from build123d import *

# Parameters (mm, degrees)
AUFSATZ_LINEAR_AUSTRAGEN1_DEPTH      = 9.8
AUFSATZ_LINEAR_AUSTRAGEN1_DEPTH_BACK = 9.8
SKIZZE1_R                            = 9.6
SKIZZE2_R                            = 11.1
AUFSATZ_LINEAR_AUSTRAGEN2_DEPTH      = 1.4
AUFSATZ_LINEAR_START                 = -1.4
SKIZZE3_R                            = 11.1
AUFSATZ_LINEAR_AUSTRAGEN3_DEPTH      = 1.4
SKIZZE4_R                            = 2
SKIZZE4_R_2                          = 3.4
SCHNITT_LINEAR_AUSTRAGEN1_DEPTH      = 1.35
KREISMUSTER1_COUNT                   = 4
SKIZZE9_R                            = 1.5
SCHNITT_LINEAR_AUSTRAGEN2_DEPTH      = 1.2


with BuildPart() as part:
    # Skizze1 → Aufsatz-Linear austragen1 (new, two sides: drawn at the far end of the back side and taken through both)
    with BuildSketch(Plane.XY.offset(-AUFSATZ_LINEAR_AUSTRAGEN1_DEPTH_BACK)):
        Circle(SKIZZE1_R)
    extrude(amount=AUFSATZ_LINEAR_AUSTRAGEN1_DEPTH + AUFSATZ_LINEAR_AUSTRAGEN1_DEPTH_BACK)

    # Skizze2 → Aufsatz-Linear austragen2 (add)
    with BuildSketch(Plane.XY.offset(9.8)):
        Circle(SKIZZE2_R)
    extrude(amount=-AUFSATZ_LINEAR_AUSTRAGEN2_DEPTH)

    # Skizze3 → Aufsatz-Linear austragen3 (add)
    with BuildSketch(Plane(origin=(0, 0, -9.8), x_dir=(-1, 0, 0), z_dir=(0, 0, -1)).offset(AUFSATZ_LINEAR_START)):
        with Locations(Location((0, 0, 0), (0, 0, 180))):
            Circle(SKIZZE3_R)
    extrude(amount=AUFSATZ_LINEAR_AUSTRAGEN3_DEPTH)

    # Skizze4 → Schnitt-Linear austragen1 (cut)
    with BuildSketch(Plane.XY.offset(9.8)):
        with Locations((0, 8.3)):
            Circle(SKIZZE4_R)
        with BuildLine():
            Line((-1.971343548, 8.637349398), (-3.351284031, 0.573493976))
            ThreePointArc((-3.351284031, 0.573493976), (0, 3.4), (3.351284031, 0.573493976))
            Line((3.351284031, 0.573493976), (1.971343548, 8.637349398))
            ThreePointArc((1.971343548, 8.637349398), (1.99282301, 8.469282167), (2, 8.3))
            ThreePointArc((2, 8.3), (-0.169282167, 6.30717699), (-1.971343548, 8.637349398))
        make_face()
        Circle(SKIZZE4_R_2)
    schnitt_linear_austragen1 = extrude(amount=-SCHNITT_LINEAR_AUSTRAGEN1_DEPTH, mode=Mode.SUBTRACT)

    # Kreismuster1: Schnitt-Linear austragen1 ×4 about axis
    kreismuster1_axis = Axis((0, 0, 0), (0, 0, 1))
    for i in range(1, KREISMUSTER1_COUNT):
        add(schnitt_linear_austragen1.rotate(kreismuster1_axis, i * 360 / KREISMUSTER1_COUNT), mode=Mode.SUBTRACT)

    # Skizze8 → Schnitt-Rotation1 (revolve, cut)
    with BuildSketch(Plane(origin=(0, 0, 0), x_dir=(0, 0, -1), z_dir=(1, 0, 0)), mode=Mode.PRIVATE) as schnitt_rotation1_sk:
        Polygon((9.8, 0), (9.8, 8), (8.4, 8), (-8.4, 3.5), (-8.4, 0), align=None)
    revolve(schnitt_rotation1_sk.sketch.rotate(Axis((0, 0, -9.8), (0, 0, 1)), 90), axis=Axis((0, 0, -9.8), (0, 0, 1)), mode=Mode.SUBTRACT)

    # Skizze9 → Schnitt-Linear austragen2 (cut)
    with BuildSketch(Plane.XY.offset(8.45)):
        Circle(SKIZZE9_R)
    extrude(amount=-SCHNITT_LINEAR_AUSTRAGEN2_DEPTH, mode=Mode.SUBTRACT)


solid = part.part
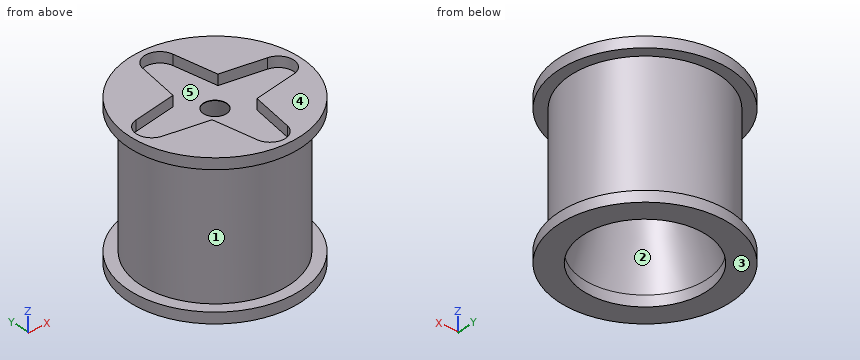
Design review of the part built by this model. Coordinates are the model's own, in mm. Face numbers are marked on the shaded views. A direction names the side the tool comes from. Round coordinates to 2 decimals unless told otherwise and drop trailing zeros. Loops run counter-clockwise (first coordinate to the right, second up) from the corner with the lowest first, then second, coordinate; pieces in that order, holes last. Notation, with made-up numbers: (14, 88.25) -> (67, 88.25) arc R15 ccw to (67, 101.25) -> close; hole circle Ø8 at (-5, 53.5). An arc over 180 degrees is marked (long way). Use one line per item in the form item = value. Start each with the question number.
Q1. We need section A-A on y = 0. Give the boundary of the cut face in (x, z).
Q2. Machinability: for the marked faces 4 and 5, which of the approach directions +Z, -Z, +X, -X, +Y, -Y give a long, thin tool a straight path to every point of the face, cutting with its end or side? Answer none if there is none.
Q3. We need section D-D on z = 0.5. Give the boundary of the cut face in (x, y), then the cut area to 3 significant figures.
Q4. Draft analysis for pull direction X (two halves, no side actions). For the marked faces 1, 2 and 3, state which applies: +X half, -X half, draft (parallel to the pull), parting line (faces both ways), or undercut.
Q5. For pin 1 Ø8 at (y, z) = (7.5, 3) entering from -X; pin 2 Ø4 at (x, z) = (-4.5, -1.5) entering from +Y; pin 3 Ø1 at (y, z) = (5, 0.5) entering from -X, all flat-tipped, find the tip position at first contact; note any pin that passes through.
Q6. We need section C-C on z = -3.25. Give the boundary of the cut face in (x, y).
Q7. Wall thickness on line 1 along Y through (x, z) = (0, -9.4); line 2 along Z through (x, y) = (6.5, -7.25); line 3 along Z through (x, y) = (-9, -0.75): over which ranges is each line inside the solid? List them lowest first. Write a range as [from, to].
Calculated:
q1.outline = (-11.1, -9.8) -> (-8, -9.8) -> (-8, -8.4) -> (-3.5, 8.4) -> (-1.5, 8.4) -> (-1.5, 8.45) -> (-10.3, 8.45) -> (-10.3, 9.8) -> (-11.1, 9.8) -> (-11.1, 8.4) -> (-9.6, 8.4) -> (-9.6, -8.4) -> (-11.1, -8.4) -> close; (1.5, 8.4) -> (3.5, 8.4) -> (8, -8.4) -> (8, -9.8) -> (11.1, -9.8) -> (11.1, -8.4) -> (9.6, -8.4) -> (9.6, 8.4) -> (11.1, 8.4) -> (11.1, 9.8) -> (10.3, 9.8) -> (10.3, 8.45) -> (1.5, 8.45) -> close
q2.face_4 = +Z, +X, -X, +Y, -Y
q2.face_5 = +Z
q3.outline = circle Ø19.2 at (0, 0); hole circle Ø11.23 at (0, 0)
q3.area = 190 mm²
q4.face_1 = parting line
q4.face_2 = undercut
q4.face_3 = draft
q5.pin_1 = -8.94
q5.pin_2 = 9.27
q5.pin_3 = -8.48
q6.outline = circle Ø19.2 at (0, 0); hole circle Ø13.24 at (0, 0)
q7.line_1 = [-11.1, -8], [8, 11.1]
q7.line_2 = [-9.8, -8.4], [8.4, 9.8]
q7.line_3 = [-9.8, 8.45]
